```python
from build123d import *

# Parameters (mm, degrees)
SKETCH1_R           = 12.7
BOSS_EXTRUDE1_DEPTH = 45
SKETCH2_R           = 10.59
BOSS_EXTRUDE2_DEPTH = 25
FILLET1_R           = 1
CHAMFER2_SIZE       = 1
CHAMFER3_SIZE       = 1


with BuildPart() as part:
    # Sketch1 → Boss-Extrude1 (new body)
    with BuildSketch(Plane.XY):
        Circle(SKETCH1_R)
    extrude(amount=BOSS_EXTRUDE1_DEPTH)

    # Sketch2 → Boss-Extrude2 (add)
    with BuildSketch(Plane(origin=(0, 0, 0), x_dir=(-1, 0, 0), z_dir=(0, 0, -1))):
        Circle(SKETCH2_R)
    extrude(amount=BOSS_EXTRUDE2_DEPTH)

    # Fillet1
    fillet1_edges = [part.edges().sort_by_distance(p)[0] for p in [
        (10.59, 0, 0),
    ]]
    fillet(fillet1_edges, radius=FILLET1_R)

    # Chamfer2
    chamfer2_edges = [part.edges().sort_by_distance(p)[0] for p in [
        (10.59, 0, -25),
    ]]
    chamfer(chamfer2_edges, length=CHAMFER2_SIZE)

    # Chamfer3
    chamfer3_edges = [part.edges().sort_by_distance(p)[0] for p in [
        (-12.7, 0, 45),
    ]]
    chamfer(chamfer3_edges, length=CHAMFER3_SIZE)


solid = part.part
```
Part model, mm, in its own coordinate system. A direction names the side the tool comes from. Give positions to 0.01 mm unless a question says otherwise; leave off trailing zeros. Order: outer loops, then holes, each group sorted by start corner. A loop starts at its lowest first (then second) coordinate and runs counter-clockwise, first axis right, second up. Notation, with made-up numbers: M 35,24.25 L 69,24.25 A13 ccw 69,41.25 Z; hole C -21.75,-30.5 d10. An arc over 180 degrees is marked long. Use a Markdown table: item, result. Add a question column.
(1) Saw through at D-D, the plane z = -6. Give the cut face in (x, y).
(2) Drop flat-ended pins along their axis: P1, Ø2, axis at y = 7, z = 2.5, coming from the +X side; P2, Ø3, axis at x = 0, z = -17.5, coming from the +Y side; P3, Ø2, axis at y = 4.5, z = -16, coming from the -X side. Give the stop position or say it passes through.
(3) 3-axis set-ups, long thin cutter, end or side, ignore diameter. For faces 1 (the face through (2.296, -10.338, -12.339)), 2 (the face through (-2.75, -12.4, 21.69)): which of +Z, -Z, +X, -X, +Y, -Y reach the whole face in a straight line?
(4) Probe line 1 along Z through (x, y) = (10.5, 4.5); line 2 along X through (y, z) = (-3.5, 5.5); line 3 along X through (y, z) = (10, 6.5). List the from-to ranges inside material, lowest first. Write a range as [from, to].
(5) Saw through at A-A, the plane x = 0. Give the cut face in (y, z).
(6) Saw through at C-C, the plane z = 27. Give the cut face in (x, y).
Answer key:
| question | item | result |
|---|---|---|
| 1 | outline | C 0,0 d21.18 |
| 2 | P1 | x = 11.19 |
| 2 | P2 | y = 10.59 |
| 2 | P3 | x = -9.99 |
| 3 | face 1 | -Z |
| 3 | face 2 | +Z, -Z |
| 4 | line 1 | [-0.01, 45] |
| 4 | line 2 | [-12.21, 12.21] |
| 4 | line 3 | [-7.83, 7.83] |
| 5 | outline | M -12.7,0 L -11.59,0 A1 cw -10.59,-1 L -10.59,-24 L -9.59,-25 L 9.59,-25 L 10.59,-24 L 10.59,-1 A1 cw 11.59,0 L 12.7,0 L 12.7,44 L 11.7,45 L -11.7,45 L -12.7,44 Z |
| 6 | outline | C 0,0 d25.4 |
